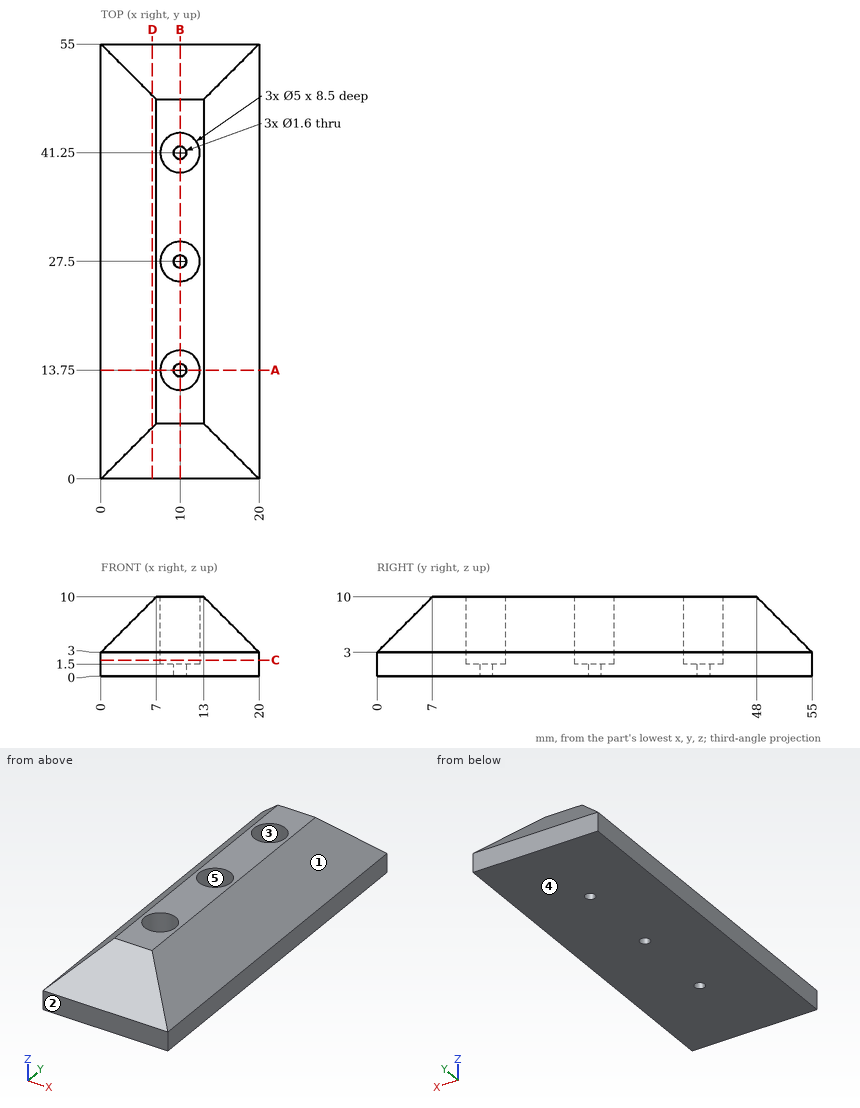
Can you work these out from the drawing? Everything is in mm from the part's minimum corner. A direction names the side the tool comes from. Give positions to 0.01 mm unless a question says otherwise; leave off trailing zeros. Order: outer loops, then holes, each group sorted by start corner. A loop starts at its lowest first (then second) coordinate and runs counter-clockwise, first axis right, second up.
1. I need wall thicknesses on L1, parallel to Y at x = 10, z = 1.2; L2, parallel to X at y = 13.75, z = 1.1; L3, parallel to Y at x = 10, z = 4. Which ranges of each line are inside material? Lowest first, please.
2. Suppose I cut it at A-A (y = 13.75). List the corners of the cut face in (x, z) for me.
3. Suppose I cut it at D-D (x = 6.5). List the corners of the cut face in (y, z) for me.
4. Suppose I cut it at C-C (z = 2). List the corners of the cut face in (x, y) for me.
5. We'd pull the mould along X, two halves only. Please class the marked faces 1, 2 and 3: pulls with the +X half, pulls with the -X half, needs draft (parallel to the pull), parting line crosses it, or undercut.
6. For the marked faces 4 and 5, which set-ups out of +Z, -Z, +X, -X, +Y, -Y let a thin tool reach every point of the face, with its end or its side?
7. Will these pins go through, and if not, where does the flat tip stop? P1, Ø2.5, axis at x = 10.5, y = 27.5, coming from the +Z side; P2, Ø1, axis at y = 32.5, z = 8, coming from the -X side.
8. Suppose I cut it at B-B (x = 10). Give the number of separate pieces and of enclosed holes in the cut face, plus the area to 3 significant figures.
Solved:
1. L1: y = 0 to 12.95, 14.55 to 26.7, 28.3 to 40.45, 42.05 to 55
1. L2: x = 0 to 9.2, 10.8 to 20
1. L3: y = 1 to 11.25, 16.25 to 25, 30 to 38.75, 43.75 to 54
2. outline: (0, 0) - (9.2, 0) - (9.2, 1.5) - (7.5, 1.5) - (7.5, 10) - (7, 10) - (0, 3) - close; (10.8, 0) - (20, 0) - (20, 3) - (13, 10) - (12.5, 10) - (12.5, 1.5) - (10.8, 1.5) - close
3. outline: (0, 0) - (55, 0) - (55, 3) - (48.5, 9.5) - (6.5, 9.5) - (0, 3) - close
4. outline: (0, 0) - (20, 0) - (20, 55) - (0, 55) - close; hole circle Ø5 at (10, 13.75); hole circle Ø5 at (10, 27.5); hole circle Ø5 at (10, 41.25)
5. face 1: pulls with the +X half
5. face 2: needs draft
5. face 3: undercut
6. face 4: -Z, +X, -X, +Y, -Y
6. face 5: +Z
7. P1: stops at z = 1.5
7. P2: stops at x = 4.5
8. separate pieces: 4
8. enclosed holes: 0
8. area: 366 mm2
